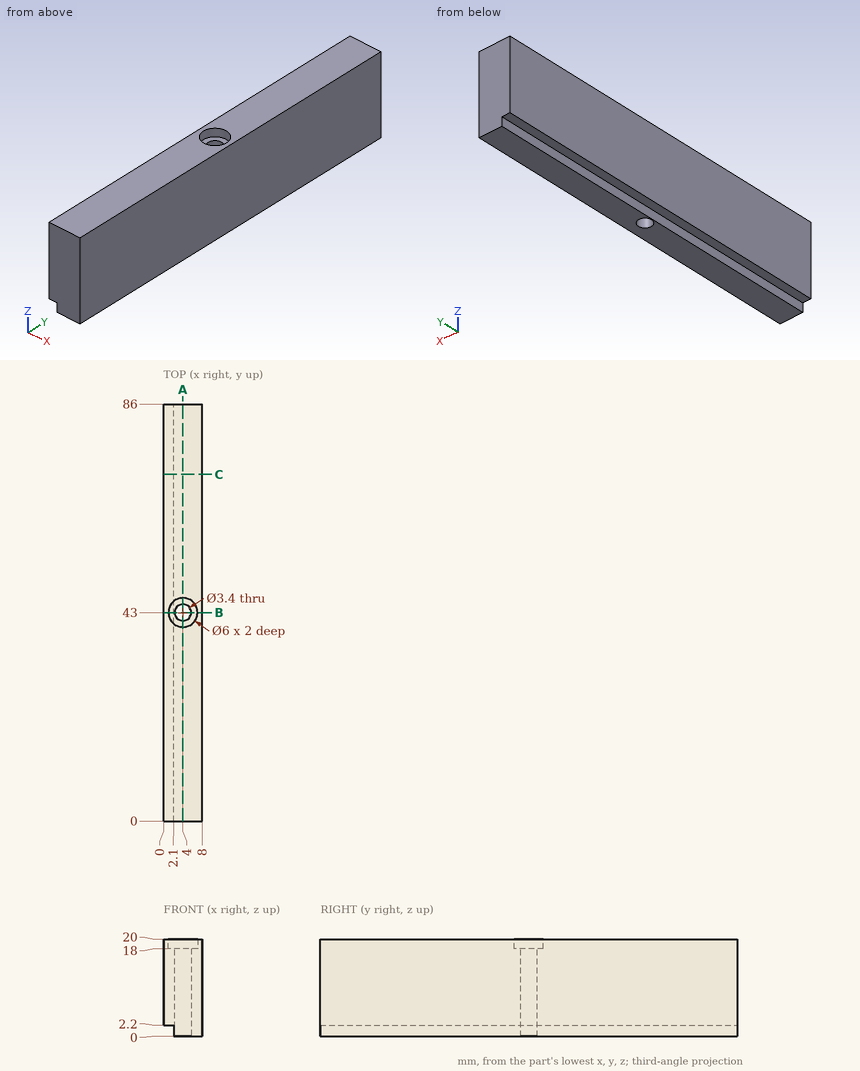
Answer from the drawing. Dimensions are ordinates in mm from the lowest x, y and z of the part. Coordinates: 2 decimals unless noted, no trailing zeros. Order: outer loops, then holes, each group sorted by start corner. A loop starts at its lowest first (then second) coordinate and runs counter-clockwise, first axis right, second up. Notation, with made-up numbers: (20, 72.5) - (65, 72.5) arc R19 cw to (65, 77.5) - close; hole circle Ø6 at (-1, -17.75). An arc over 180 degrees is marked (long way). Put each result on its own line as item: value. Start each with the question number.
1) Flat-ended cylindrical pins translate along their axes: pin 1 (3 mm diameter, centred on x = 2.5, z = 17, fed in from -Y); pin 2 (0.7 mm diameter, centred on y = 64.5, z = 0.5, fed in from -X); pin 3 (1.7 mm diameter, centred on x = 1, y = 25, fed in from -Z). Find the tip coordinate at first contact, or state that the pin passes through.
2) Find the intervals of material crossed by line 1 (Y direction, x = 4, z = 14); line 2 (Z direction, x = 1, y = 60); line 3 (Y direction, x = 5.25, z = 2.75), in increasing order. Write a range as from..to.
3) Find section C-C (y = 71.5). Give the vertices of the cut face in (x, z).
4) Find section A-A (x = 4). Give the vertices of the cut face in (y, z), plus the area to 3 significant figures.
5) Find section B-B (y = 43). Give the vertices of the cut face in (x, z), plus the area to 3 significant figures.
Results list:
1. pin 1: stops at y = 0
1. pin 2: stops at x = 2.1
1. pin 3: stops at z = 2.2
2. line 1: y = 0..41.3, 44.7..86
2. line 2: z = 2.2..20
2. line 3: y = 0..41.85, 44.15..86
3. outline: (0, 2.2) - (2.1, 2.2) - (2.1, 0) - (8, 0) - (8, 20) - (0, 20) - close
4. outline: (0, 0) - (41.3, 0) - (41.3, 18) - (40, 18) - (40, 20) - (0, 20) - close; (44.7, 0) - (86, 0) - (86, 20) - (46, 20) - (46, 18) - (44.7, 18) - close
4. area: 1,650 mm^2
5. outline: (0, 2.2) - (2.1, 2.2) - (2.1, 0) - (2.3, 0) - (2.3, 18) - (1, 18) - (1, 20) - (0, 20) - close; (5.7, 0) - (8, 0) - (8, 20) - (7, 20) - (7, 18) - (5.7, 18) - close
5. area: 82.2 mm^2
